Could you check a few things on this model? Use its own coordinates, in mm. Face numbers are marked on the shaded views. Give positions to 0.01 mm unless a question says otherwise; leave off trailing zeros. Write each loop counter-clockwise with the first axis right and the second up, starting at its lowest first coordinate (ties: lowest second). Pieces come first, ordered by that corner, then holes. Notation, with made-up numbers: (-5.5, -37.5) - (50.5, -37.5) arc R16 cw to (50.5, -17.5) - close; hole circle Ø6 at (38.5, 46.25). An arc over 180 degrees is marked (long way). Answer in a Markdown table with one row per item.
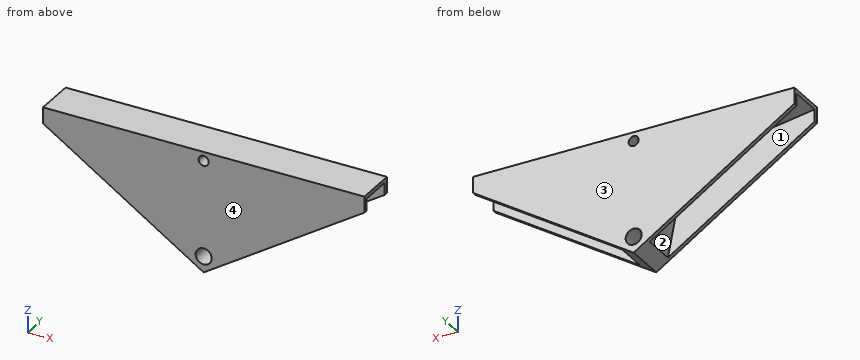
from build123d import *

# Parameters (mm, degrees)
SKETCH1_R           = 2
SKETCH1_R_2         = 1.25
BOSS_EXTRUDE1_DEPTH = 10
CUT_EXTRUDE1_DEPTH  = 8


with BuildPart() as part:
    # Sketch1 → Boss-Extrude1 (new body)
    with BuildSketch(Plane(origin=(0, 0, 0), x_dir=(1, 0, 0), z_dir=(0, 1, 0))):
        Polygon((0, 26), (-40, 0), (-40, -4), (40, -4), (40, 0), align=None)
        with Locations((0, 22)):
            Circle(SKETCH1_R, mode=Mode.SUBTRACT)
        with Locations((0, -1.8)):
            Circle(SKETCH1_R_2, mode=Mode.SUBTRACT)
    extrude(amount=BOSS_EXTRUDE1_DEPTH)

    # Sketch2 → Cut-Extrude1 (cut)
    with BuildSketch(Plane(origin=(0, 9, 0), x_dir=(1, 0, 0), z_dir=(0, 1, 0))):
        Polygon((-3, 26), (-7.746877636, 2), (-40, -3), (-40, 3.063809347), align=None)
    cut_extrude1 = extrude(amount=-CUT_EXTRUDE1_DEPTH, mode=Mode.SUBTRACT)

    # Mirror1: Cut-Extrude1 across plane
    add(cut_extrude1.mirror(Plane(origin=(0, 0, 0), x_dir=(0, 0, 1), z_dir=(1, 0, 0))), mode=Mode.SUBTRACT)


solid = part.part
1) If I drill on line 1 (Z direction, x = 0, y = 3); line 2 (Y direction, x = -9, z = -2); line 3 (X direction, y = 2.5, z = -22), over which ranges is the centre line in solid material (lowest first)?
Check values:
| item | result |
|---|---|
| line 1 | z = -26 to -24, -20 to 0.55, 3.05 to 4 |
| line 2 | y = 0 to 1, 9 to 10 |
| line 3 | x = -3.79 to -2, 2 to 3.79 |
2) We'd pull the mould along Y, two halves only. Please class the marked faces 1, 2, 3 and 4: +Y half, -Y half, draft (parallel to the pull), parting line (faces both ways), or undercut.
Check values:
| item | result |
|---|---|
| face 1 | undercut |
| face 2 | undercut |
| face 3 | +Y half |
| face 4 | -Y half |
3) Imagine slicing it at A-A (z = -21). List the corners of the cut face in (x, y) for me.
Check values:
| item | result |
|---|---|
| outline | (-7.69, 0) - (-1.73, 0) - (-1.73, 10) - (-7.69, 10) - (-7.69, 9) - (-3.99, 9) - (-3.99, 1) - (-7.69, 1) - close; (1.73, 0) - (7.69, 0) - (7.69, 1) - (3.99, 1) - (3.99, 9) - (7.69, 9) - (7.69, 10) - (1.73, 10) - close |
4) Imagine slicing it at B-B (y = 7.25). List the corners of the cut face in (x, z) for me, then the cut area to 3 significant figures.
Check values:
| item | result |
|---|---|
| outline | (-40, 3) - (-7.75, -2) - (-3.44, -23.76) - (0, -26) - (3.44, -23.76) - (7.75, -2) - (40, 3) - (40, 4) - (-40, 4) - close; hole circle Ø4 at (0, -22); hole circle Ø2.5 at (0, 1.8) |
| area | 552 mm2 |
5) Will these pins go through, and if not, where does the flat tip stop? P1, Ø1, axis at y = 7.5, z = -14, coming from the -X side; P2, Ø2, axis at x = -18, y = 6, coming from the -Z side; P3, Ø4, axis at y = 3.5, z = -14.5, coming from the +X side; P4, Ø2.5, axis at x = 0, z = -22, coming from the +Y side.
Check values:
| item | result |
|---|---|
| P1 | stops at x = -5.47 |
| P2 | stops at z = -0.57 |
| P3 | stops at x = 5.67 |
| P4 | passes through |
6) Imagine slicing it at D-D (z = 1.8). List the corners of the cut face in (x, y) for me, then the cut area to 3 significant figures.
Check values:
| item | result |
|---|---|
| outline | (-40, 0) - (-1.25, 0) - (-1.25, 10) - (-40, 10) - (-40, 9) - (-32.26, 9) - (-32.26, 1) - (-40, 1) - close; (1.25, 0) - (40, 0) - (40, 1) - (32.26, 1) - (32.26, 9) - (40, 9) - (40, 10) - (1.25, 10) - close |
| area | 651 mm2 |
7) Imagine slicing it at C-C (x = -6.5). List the corners of the cut face in (y, z) for me (3 decimals), then the cut area to 3 significant figures.
Check values:
| item | result |
|---|---|
| outline | (0, -21.775) - (1, -21.775) - (1, -8.304) - (9, -8.304) - (9, -21.775) - (10, -21.775) - (10, 4) - (0, 4) - close |
| area | 150 mm2 |
